Design review of the part built by this model. Coordinates are the model's own, in mm. A direction names the side the tool comes from. Coordinates: 2 decimals unless noted, no trailing zeros. Write each loop counter-clockwise with the first axis right and the second up, starting at its lowest first coordinate (ties: lowest second). Pieces come first, ordered by that corner, then holes.
Q1. Clearance check with a flat-ended pin moving along its axis: pin 1 Ø0.5 at (x, z) = (33.5, 1) entering from +Y. State where the tip first meets the part, or that it passes through.
Q2. The part is to be moulded in two halves that separate along Y. For faces 3 (the face through (108.28, 47.22, 0.91)), 4 (the face through (103.358, -15.199, 0.887)), 5 (the face through (50, -4, 1.8)), say which applies: +Y half, -Y half, draft (parallel to the pull), parting line (faces both ways), or undercut.
Q3. To check wall thickness, follow probe 1 along X at (y, z) = (28, 0.3); probe 2 along X at (y, z) = (-1, 1.6); probe 3 along Y at (x, z) = (39, 1.25). State the ranges of each line that lie inside material, in increasing order.
Q4. Add section C-C, the plane x = -14.5. Give the boundary of the cut face in (y, z).
Q5. Machinability: for faces 1 (the face through (106.02, 15, 0.91)), 2 (the face through (-21.22, 47.17, 0.91)), which of the approach directions +Z, -Z, +X, -X, +Y, -Y give a long, thin tool a straight path to every point of the face, cutting with its end or side? Answer none if there is none.
Q6. Add section B-B, the plane z = 0.9. Give the number of separate pieces and of enclosed holes in the cut face, plus the area to 3 significant figures.
Q7. Add section A-A, the plane y = 33.5. Give the boundary of the cut face in (x, z).
Q8. Add section D-D, the plane y = -15.8. Give the boundary of the cut face in (x, z), plus the area to 3 significant figures.
from build123d import *

# Parameters (mm, degrees)
SKETCH_1_R      = 1.5
SKETCH_1_R_2    = 2
EXTRUDE_1_DEPTH = 1.8
FILLET_1_R      = 2.75
FILLET_2_R      = 5


with BuildPart() as part:
    # 草图1 → 凸台-拉伸1 (new body)
    with BuildSketch(Plane.XY):
        Polygon((-22, -24.8), (109.95, -24.8), (123.45, 11), (123.45, 48), (107.45, 48), (107.45, 13.5), (-6, 13.5), (-6, 48), (-22, 48), align=None)
        Circle(SKETCH_1_R, mode=Mode.SUBTRACT)
        with Locations((107.45, 0)):
            Circle(SKETCH_1_R, mode=Mode.SUBTRACT)
        with Locations((115.45, 20)):
            Circle(SKETCH_1_R_2, mode=Mode.SUBTRACT)
        with Locations((-14, 20)):
            Circle(SKETCH_1_R_2, mode=Mode.SUBTRACT)
        with Locations((-14.5, -15.8)):
            Circle(SKETCH_1_R_2, mode=Mode.SUBTRACT)
        with Locations((101.45, -15.8)):
            Circle(SKETCH_1_R_2, mode=Mode.SUBTRACT)
        with Locations((115.45, 44)):
            Circle(SKETCH_1_R_2, mode=Mode.SUBTRACT)
        with Locations((-14, 44)):
            Circle(SKETCH_1_R_2, mode=Mode.SUBTRACT)
        with Locations((53.725, 7)):
            Circle(SKETCH_1_R_2, mode=Mode.SUBTRACT)
        with Locations(Location((53.725, -7, 0), (0, 0, 180))):
            Circle(SKETCH_1_R_2, mode=Mode.SUBTRACT)
    extrude(amount=EXTRUDE_1_DEPTH)

    # 圆角1
    fillet_1_edges = [part.edges().sort_by_distance(p)[0] for p in [
        (-22, 48, 0.9),
        (-6, 48, 0.9),
        (107.45, 48, 0.9),
        (123.45, 48, 0.9),
        (-22, -24.8, 0.9),
    ]]
    fillet(fillet_1_edges, radius=FILLET_1_R)

    # 圆角2
    fillet_2_edges = [part.edges().sort_by_distance(p)[0] for p in [
        (-6, 13.5, 0.9),
        (107.45, 13.5, 0.9),
    ]]
    fillet(fillet_2_edges, radius=FILLET_2_R)


solid = part.part
Here are the results:
1. pin 1: stops at y = 13.5
2. face 3: +Y half
2. face 4: undercut
2. face 5: draft
3. probe 1: x = -22 to -6, 107.45 to 123.45
3. probe 2: x = -22 to -1.12, 1.12 to 106.33, 108.57 to 118.92
3. probe 3: y = -24.8 to 13.5
4. outline: (-24.8, 0) - (-17.8, 0) - (-17.8, 1.8) - (-24.8, 1.8) - close; (-13.8, 0) - (18.06, 0) - (18.06, 1.8) - (-13.8, 1.8) - close; (21.94, 0) - (42.06, 0) - (42.06, 1.8) - (21.94, 1.8) - close; (45.94, 0) - (48, 0) - (48, 1.8) - (45.94, 1.8) - close
5. face 1: +Z, -Z, +Y
5. face 2: +Z, -Z, -X, +Y
6. separate pieces: 1
6. enclosed holes: 10
6. area: 6,320 mm2
7. outline: (-22, 0) - (-6, 0) - (-6, 1.8) - (-22, 1.8) - close; (107.45, 0) - (123.45, 0) - (123.45, 1.8) - (107.45, 1.8) - close
8. outline: (-22, 0) - (-16.5, 0) - (-16.5, 1.8) - (-22, 1.8) - close; (-12.5, 0) - (99.45, 0) - (99.45, 1.8) - (-12.5, 1.8) - close; (103.45, 0) - (113.34, 0) - (113.34, 1.8) - (103.45, 1.8) - close
8. area: 229 mm2
